Check sheet for the drawn part. Datum: minimum x, y, z corner. Units: mm. A direction names the side the tool comes from. Round coordinates to 2 decimals unless told otherwise and drop trailing zeros. Loops run counter-clockwise (first coordinate to the right, second up) from the corner with the lowest first, then second, coordinate; pieces in that order, holes last.
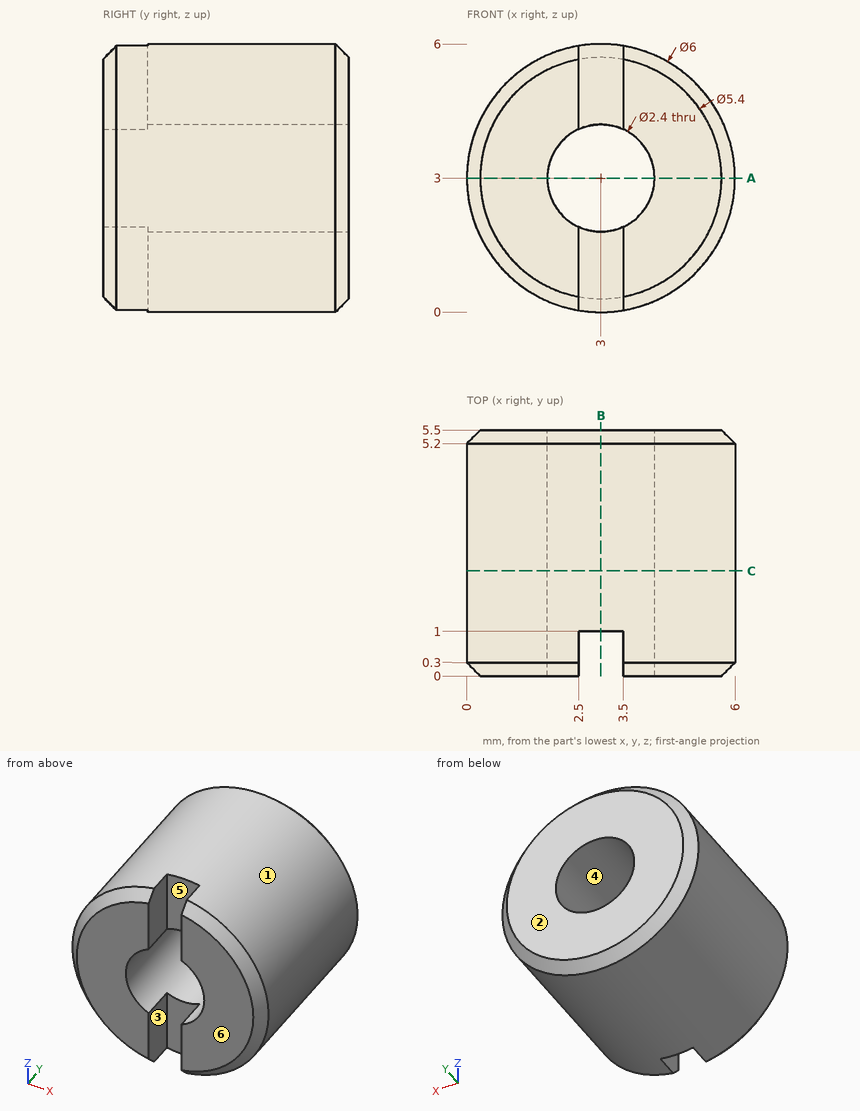
1) Sectioned sample at A-A, the plane z = 3. Record the cut outline in (x, y), then the cut area to 3 significant figures.
Report:
outline: (0, 0.3) - (0.3, 0) - (1.8, 0) - (1.8, 5.5) - (0.3, 5.5) - (0, 5.2) - close; (4.2, 0) - (5.7, 0) - (6, 0.3) - (6, 5.2) - (5.7, 5.5) - (4.2, 5.5) - close
area: 19.6 mm2
2) Sectioned sample at B-B, the plane x = 3. Record the cut outline in (y, z), then the cut area to 3 significant figures.
Report:
outline: (1, 0) - (5.2, 0) - (5.5, 0.3) - (5.5, 1.8) - (1, 1.8) - close; (1, 4.2) - (5.5, 4.2) - (5.5, 5.7) - (5.2, 6) - (1, 6) - close
area: 16.1 mm2
3) Mould release check, pull along X, two halves, no side actions. Record for the marked faces 1, 2, 3 and 4: +X half, -X half, draft (parallel to the pull), parting line (faces both ways), or undercut.
Report:
face 1: parting line
face 2: draft
face 3: undercut
face 4: undercut
4) Access from +Z, -Z, +X, -X, +Y, -Y to the whole of each face (thin tool, end or side, straight path). Record for the marked faces 5 and 6.
Report:
face 5: +Z, -Z, -Y
face 6: +Z, -Z, +X, -X, -Y
5) Gauge pin test, flat ends, axial feed: pin 1 (0.8 mm diameter, centred on y = 0.5, z = 0.5, fed in from +X); pin 2 (0.8 mm diameter, centred on x = 3, z = 5, fed in from -Y); pin 3 (0.8 mm diameter, centred on y = 0.5, z = 4.5, fed in from -X); pin 4 (1.5 mm diameter, centred on x = 4, z = 3.5, fed in from +Y). Record the tip position at first contact, or that the pin passes through.
Report:
pin 1: stops at x = 5.14
pin 2: stops at y = 1
pin 3: stops at x = 0.21
pin 4: stops at y = 5.5
6) Scan lines: line 1 along Z through (x, y) = (3, 3.7); line 2 along Z through (x, y) = (4, 2.05); line 3 along X through (y, z) = (2.55, 5.75). Record each from-to range of solid material in increasing order.
Report:
line 1: z = 0 to 1.8, 4.2 to 6
line 2: z = 0.17 to 2.34, 3.66 to 5.83
line 3: x = 1.8 to 4.2
7) Sectioned sample at C-C, the plane y = 2.35. Record the cut outline in (x, z).
Report:
outline: circle Ø6 at (3, 3); hole circle Ø2.4 at (3, 3)
